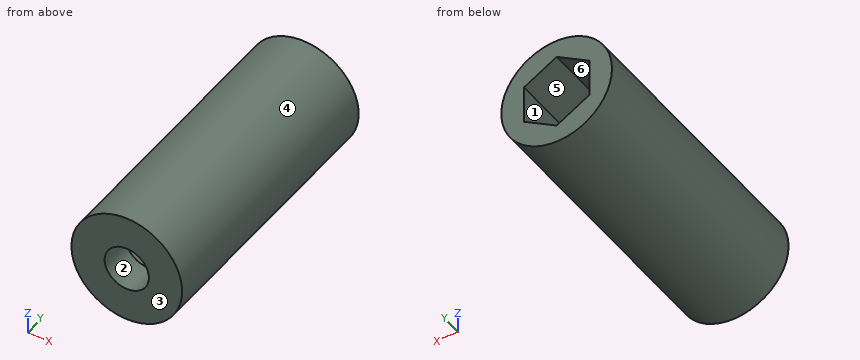
Autodesk Inventor part; units mm, degrees
ref_plane "YZ Plane" through (0, 0, 0) normal (1, 0, 0) x (0, 1, 0)
ref_plane "XZ Plane" through (0, 0, 0) normal (0, 1, 0) x (-1, 0, 0)
ref_plane "XY Plane" through (0, 0, 0) normal (0, 0, 1) x (1, 0, 0)
sketch "草图1" plane through (0, 0, 0) normal (0, 1, 0) x (-1, 0, 0)
  circle A0 centre (0, 0) radius 5
  line L0 (2.95, -1.7032) -> (0, -3.4064)
  line L1 (0, -3.4064) -> (-2.95, -1.7032)
  line L2 (-2.95, -1.7032) -> (-2.95, 1.7032)
  line L3 (-2.95, 1.7032) -> (0, 3.4064)
  line L4 (0, 3.4064) -> (2.95, 1.7032)
  line L5 (2.95, 1.7032) -> (2.95, -1.7032)
  point P0 (2.95, 0)
  dimension "d0" = 10
extrude "拉伸1" add sketch "草图1" along normal blind 25
sketch "草图3" plane through (0, 0, 0) normal (0, -1, 0) x (1, 0, 0)
  circle A0 centre (0, 0) radius 2
  circle A1 centre (0, 0) radius 5
  dimension "d7" = 4
extrude "拉伸3" add sketch "草图3" against normal blind 3
properties part number "机械爪六角筒"
Source: CAD feature listing. Evaluate the final solid. Frame: model axes, mm. Face numbers are marked on the shaded views. A direction names the side the tool comes from. Coordinates: 2 decimals unless noted, no trailing zeros. Write each loop counter-clockwise with the first axis right and the second up, starting at its lowest first coordinate (ties: lowest second). Pieces come first, ordered by that corner, then holes. Notation, with made-up numbers: M 69,-34.5 L 93,-34.5 A28 cw 93,3.5 Z; hole C -0.5,-12.75 d11. An arc over 180 degrees is marked long. Use a Markdown table: item, result.
1) Ray query, L1, parallel to Z at x = 0, y = 2.2; L2, parallel to Y at x = 1.5, z = -1.5; L3, parallel to X at y = 11.25, z = -0.5. Return the intervals inside material, ascending.
Conclusion:
| item | result |
|---|---|
| L1 | z = -5 to -2, 2 to 5 |
| L2 | y = 0 to 3 |
| L3 | x = -4.97 to -2.95, 2.95 to 4.97 |
2) First-contact query: pin 1 Ø3 at (x, z) = (0, -1.5) entering from +Y; pin 2 Ø3 at (x, y) = (3.5, 11) entering from -Z. Flat tips, straight axial feed; report the tip coordinate or a pass-through.
Conclusion:
| item | result |
|---|---|
| pin 1 | stops at y = 3 |
| pin 2 | stops at z = -4.58 |
3) Section B-B, the plane z = 0. Output: boundary loops of the cut face in (x, y).
Conclusion:
| item | result |
|---|---|
| outline | M -5,0 L -2,0 L -2,3 L -2.95,3 L -2.95,25 L -5,25 Z; M 2,0 L 5,0 L 5,25 L 2.95,25 L 2.95,3 L 2,3 Z |
4) Section A-A, the plane y = 14. Output: boundary loops of the cut face in (x, z).
Conclusion:
| item | result |
|---|---|
| outline | C 0,0 d10; hole M -2.95,-1.7 L 0,-3.41 L 2.95,-1.7 L 2.95,1.7 L 0,3.41 L -2.95,1.7 Z |
5) Section C-C, the plane x = -1.75. Output: boundary loops of the cut face in (y, z), then the cut area to 3 significant figures.
Conclusion:
| item | result |
|---|---|
| outline | M 0,-4.68 L 25,-4.68 L 25,-2.4 L 3,-2.4 L 3,-0.97 L 0,-0.97 Z; M 0,0.97 L 3,0.97 L 3,2.4 L 25,2.4 L 25,4.68 L 0,4.68 Z |
| area | 123 mm^2 |
6) Mould query, pull axis X, two halves, no side actions, for the marked faces 3, 4, 5 and 6. Classes: pulls with the +X half, pulls with the -X half, needs draft (parallel to the pull), parting line crosses it, or undercut.
Conclusion:
| item | result |
|---|---|
| face 3 | needs draft |
| face 4 | parting line crosses it |
| face 5 | undercut |
| face 6 | undercut |
7) Section D-D, the plane z = 2.25. Output: boundary loops of the cut face in (x, y).
Conclusion:
| item | result |
|---|---|
| outline | M -4.47,0 L 4.47,0 L 4.47,25 L 2,25 L 2,3 L -2,3 L -2,25 L -4.47,25 Z |
8) Reachability of the marked faces 1 and 2 from +Z, -Z, +X, -X, +Y, -Y: full face, straight path, thin tool, end or side. Return the list, or none.
Conclusion:
| item | result |
|---|---|
| face 1 | +Y |
| face 2 | +Y, -Y |
